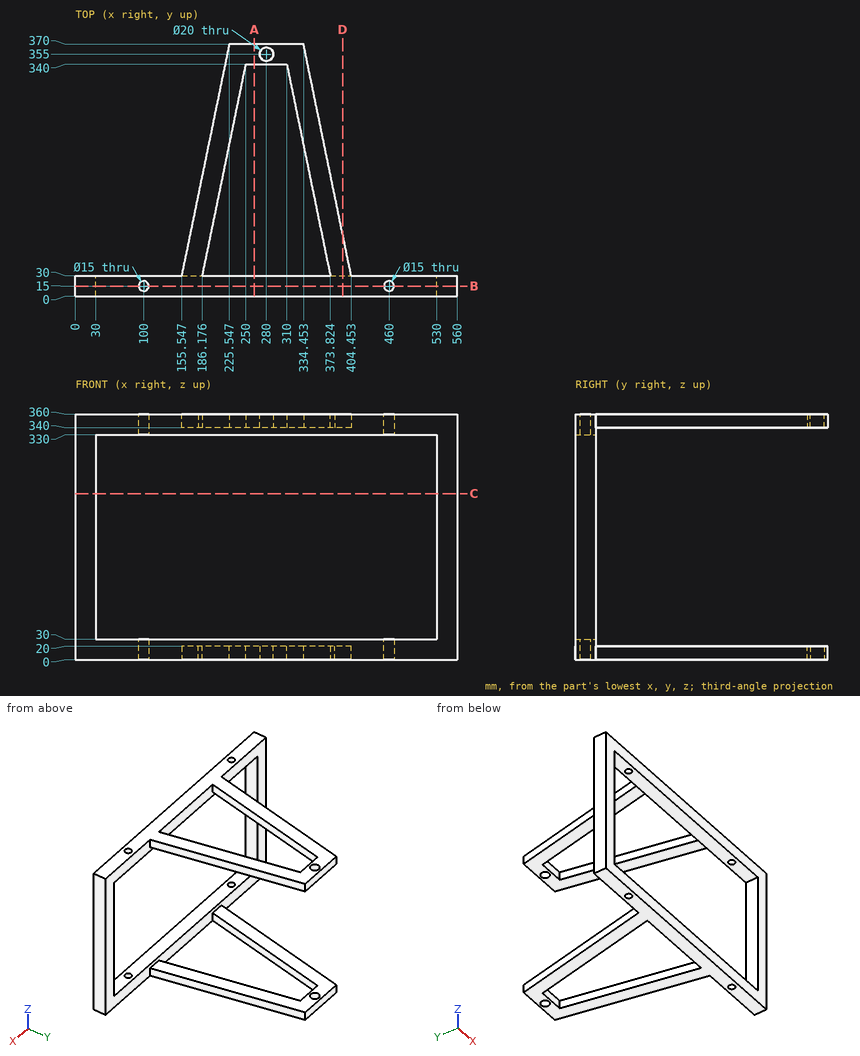
Input: dimensioned drawing with shaded views. Units: mm. Origin: part minimum x, y, z. Give positions to 0.01 mm unless a question says otherwise; leave off trailing zeros. Loops run counter-clockwise (first coordinate to the right, second up) from the corner with the lowest first, then second, coordinate; pieces in that order, holes last. Notation, with made-up numbers: (-33, -33) - (11, -33) arc R18 ccw to (11, -27) - close; hole circle Ø3 at (29.25, 38.25). An arc over 180 degrees is marked (long way). Answer as CSV lines item,"result". Start each with the question number.
(1) Pin query (flat end, axial travel): P1, Ø18, axis at x = 280, y = 355, coming from the +Z side. Return the tip coordinate at first contact, or that it passes through.
(2) Section query D-D (x = 392). Output: boundary loops of the cut face in (y, z) (1 decimal), and give its area (3 significant figures).
(3) Section query B-B (y = 15). Output: boundary loops of the cut face in (x, z), and give its area (3 significant figures).
(4) Section query C-C (z = 243.5). Output: boundary loops of the cut face in (x, y), and give its area (3 significant figures).
(5) Ray query, line 1 along Y through (x, z) = (100, 8.75); line 2 along Y through (x, z) = (280, 350); line 3 along X through (y, z) = (17, 336). Return the intervals inside material, ascending. Write a range as [from, to].
(6) Section query A-A (x = 262.5). Output: boundary loops of the cut face in (y, z), and give its area (3 significant figures).
Worked answers:
1,P1,"passes through"
2,outline,"(0, 0) - (90.5, 0) - (90.5, 20) - (30, 20) - (30, 30) - (0, 30) - close; (0, 330) - (30, 330) - (30, 340) - (90.5, 340) - (90.5, 360) - (0, 360) - close"
2,area,"4,220 mm^2"
3,outline,"(0, 0) - (92.5, 0) - (92.5, 30) - (30, 30) - (30, 330) - (92.5, 330) - (92.5, 360) - (0, 360) - close; (107.5, 0) - (452.5, 0) - (452.5, 30) - (107.5, 30) - close; (107.5, 330) - (452.5, 330) - (452.5, 360) - (107.5, 360) - close; (467.5, 0) - (560, 0) - (560, 360) - (467.5, 360) - (467.5, 330) - (530, 330) - (530, 30) - (467.5, 30) - close"
3,area,"49,800 mm^2"
4,outline,"(0, 0) - (30, 0) - (30, 30) - (0, 30) - close; (530, 0) - (560, 0) - (560, 30) - (530, 30) - close"
4,area,"1,800 mm^2"
5,line 1,"y = [0, 7.5], [22.5, 30]"
5,line 2,"y = [0, 30], [340, 345], [365, 370]"
5,line 3,"x = [0, 92.77], [107.23, 452.77], [467.23, 560]"
6,outline,"(0, 0) - (30, 0) - (30, 30) - (0, 30) - close; (0, 330) - (30, 330) - (30, 360) - (0, 360) - close; (340, 0) - (370, 0) - (370, 20) - (340, 20) - close; (340, 340) - (370, 340) - (370, 360) - (340, 360) - close"
6,area,"3,000 mm^2"
